Autodesk Inventor part; units mm, degrees
ref_plane "YZ Plane" through (0, 0, 0) normal (1, 0, 0) x (0, 1, 0)
ref_plane "XZ Plane" through (0, 0, 0) normal (0, 1, 0) x (-1, 0, 0)
ref_plane "XY Plane" through (0, 0, 0) normal (0, 0, 1) x (1, 0, 0)
sketch "草圖1" plane through (0, 0, 0) normal (0, 1, 0) x (-1, 0, 0)
  line L0 (12.03, 0) -> (-14.43, 0)
  line L1 (5.25, 0) -> (-10.4678, 0)
  line L2 (-10.65, 2.5) -> (-10.65, 16)
  line L3 (-10.65, 16) -> (5.25, 16)
  line L4 (5.25, 16) -> (5.25, 0)
  line L5 (5.25, 14.5) -> (8.25, 14.5)
  line L6 (8.25, 14.5) -> (8.25, 4.5)
  line L7 (8.25, 4.5) -> (5.25, 4.5)
  line L8 (5.25, 4.5) -> (5.25, 14.5)
  line L9 (1.5, 16) -> (-1.5, 16)
  line L10 (-1.5, 16) -> (-1.5, 12)
  line L11 (-1.5, 12) -> (1.5, 12)
  line L12 (1.5, 12) -> (1.5, 16)
  line L13 (0, -23.6) -> (0, 22.6)
  line L14 (2.75, 12) -> (-2.75, 12)
  line L15 (-2.75, 12) -> (-2.75, 9.5)
  line L16 (-2.75, 9.5) -> (2.75, 9.5)
  line L17 (2.75, 9.5) -> (2.75, 12)
  line L18 (1.5, 9.5) -> (-1.5, 9.5)
  line L19 (-1.5, 9.5) -> (-1.5, 7.5)
  line L20 (-1.5, 7.5) -> (1.5, 7.5)
  line L21 (1.5, 7.5) -> (1.5, 9.5)
  line L22 (-10.65, 16) -> (-3.65, 16)
  line L23 (-3.65, 16) -> (-3.65, -11)
  circle A0 centre (-3.65, -11) radius 1.3
  circle A1 centre (-3.65, -11) radius 6
  line L24 (5.25, 0) -> (2.1747, -12.4399)
  line L25 (-10.65, 16) -> (-10.65, 2.5)
  line L26 (-10.65, 2.5) -> (-9.6341, -11.4362)
  dimension "d0" = 16
  dimension "d1" = 15.9
  dimension "d2" = 3
  dimension "d3" = 10
  dimension "d4" = 1.5
  dimension "d5" = 1.5
  dimension "d6" = 3
  dimension "d7" = 4
  dimension "d8" = 2.5
  dimension "d9" = 1.25
  dimension "d10" = 1.25
  dimension "d11" = 1.5
  dimension "d12" = 3
  dimension "d13" = 2
  dimension "d14" = 9.15
  dimension "d15" = 7
  dimension "d16" = 27
  dimension "d17" = 2.6
  dimension "d18" = 12
  dimension "d19" = 13.5
extrude "擠出1" add sketch "草圖1" along normal mid plane 3 contours L24 A1 L13 L0 | L0 L13 L20 L21 L16 L17 L14 L12 L3 L4 | L13 A1 L23 L0 | L0 L23 L3 L10 L14 L15 L16 L19 L20 L13 | L4 L5 L6 L7 | A1 L13 | L23 A1 L26 L0 | L0 L26 L2 L3 L23 | L13 A1
properties part number "板子8"
Work out the finished part from the listing and answer in its coordinate system (mm). A direction names the side the tool comes from. Round coordinates to 2 decimals unless told otherwise and drop trailing zeros. Order: outer loops, then holes, each group sorted by start corner. A loop starts at its lowest first (then second) coordinate and runs counter-clockwise, first axis right, second up. Notation, with made-up numbers: M 45,56 L 51,56 A28 ccw 51,86 Z; hole C -39.75,5.5 d9. An arc over 180 degrees is marked long. Put each result on its own line as item: value. Start each with the question number.
Q1. Flat-ended cylindrical pins translate along their axes: pin 1 (0.6 mm diameter, centred on x = 2, y = 0, fed in from -Z); pin 2 (0.6 mm diameter, centred on x = -2, y = 0.5, fed in from -Z); pin 3 (1 mm diameter, centred on y = 0.5, z = -13.5, fed in from -X). Find the tip coordinate at first contact, or state that the pin passes through.
Q2. Section B-B, the plane z = 10 is taken. Write down the section's boundary in (x, y), and give its area (3 significant figures).
Q3. Section D-D, the plane z = 3.5 is taken. Write down the section's boundary in (x, y).
Q4. A tool of negligible diameter and unlimited length cuts with its end or side. For faces 4 (the flat face through (1.5, 0, 9)), 5 (the flat face through (-5.25, 0, 2)), 6 (the flat face through (-2.75, 0, 11)), from which of +Z, -Z, +X, -X, +Y, -Y can it reach the whole face along a straight path? Write none if from no direction.
Q5. For a pull along Z with two mould halves and no side action, classify faces 1 (the flat face through (-7, 0, 14.5)), 2 (the flat face through (-3.734, -0.021, -6.133)), 3 (the flat face through (-2, 0, 9.5)) as pulls with the +Z half, pulls with the -Z half, needs draft (parallel to the pull), parting line crosses it, or undercut.
Q6. Section C-C, the plane y = 0.6 is taken. Write down the section's boundary in (x, z), and give its area (3 significant figures).
Q7. Section A-A, the plane x = 3.65 is taken. Write down the section's boundary in (y, z), and give its area (3 significant figures).
Q8. Straight lines are drawn through the part: L1, parallel to Z at x = 3.65, y = 0.3; L2, parallel to X at y = -1.2, z = 14; L3, parallel to X at y = 0.3, z = -11. For each, find the intervals that lie inside material, in ascending order. Write a range as [from, to].
Findings below:
1. pin 1: stops at z = -16.85
1. pin 2: stops at z = -13.72
1. pin 3: stops at x = -2.01
2. outline: M -8.25,-1.5 L -2.75,-1.5 L -2.75,1.5 L -8.25,1.5 Z; M 2.75,-1.5 L 10.65,-1.5 L 10.65,1.5 L 2.75,1.5 Z
2. area: 40.2 mm^2
3. outline: M -5.25,-1.5 L 10.65,-1.5 L 10.65,1.5 L -5.25,1.5 Z
4. face 4: +Z, +Y, -Y
4. face 5: -Z, -X, +Y, -Y
4. face 6: +Y, -Y
5. face 1: pulls with the +Z half
5. face 2: pulls with the -Z half
5. face 3: undercut
6. outline: M -8.25,4.5 L -5.25,4.5 L -5.25,0 L -2.17,-12.44 A6 ccw 9.63,-11.44 L 10.65,2.5 L 10.65,16 L 1.5,16 L 1.5,12 L 2.75,12 L 2.75,9.5 L 1.5,9.5 L 1.5,7.5 L -1.5,7.5 L -1.5,9.5 L -2.75,9.5 L -2.75,12 L -1.5,12 L -1.5,16 L -5.25,16 L -5.25,14.5 L -8.25,14.5 Z; hole C 3.65,-11 d2.6
6. area: 457 mm^2
7. outline: M -1.5,-17 L 1.5,-17 L 1.5,-12.3 L -1.5,-12.3 Z; M -1.5,-9.7 L 1.5,-9.7 L 1.5,16 L -1.5,16 Z
7. area: 91.2 mm^2
8. L1: z = [-17, -12.3], [-9.7, 16]
8. L2: x = [-8.25, -1.5], [1.5, 10.65]
8. L3: x = [-2.53, 2.35], [4.95, 9.67]
